Source: CAD feature listing. Evaluate the final solid. Frame: model axes, mm. A direction names the side the tool comes from. Give positions to 0.01 mm unless a question says otherwise; leave off trailing zeros. Order: outer loops, then holes, each group sorted by start corner. A loop starts at its lowest first (then second) coordinate and runs counter-clockwise, first axis right, second up. Notation, with made-up numbers: M 78,6.5 L 90,6.5 A17 cw 90,23.5 Z; hole C 82.25,-34 d2. An arc over 180 degrees is marked long. Answer as a JSON object with one key per item and string values. Group by question number.
1. Pull-direction query (Z, two-part tool) for faces 1 (the flat face through (21, -3, 6)), 2 (the flat face through (-12.5, -3, -28)), 3 (the flat face through (25, -3, 21)); classes: +Z half, -Z half, draft (parallel to the pull), parting line (faces both ways), or undercut.
2. Pin query (flat end, axial travel): P1, Ø3, axis at y = -3.5, z = -26.5, coming from the -X side; P2, Ø3, axis at x = -5.5, y = -2, coming from the -Z side; P3, Ø1.9, axis at x = 24.75, z = 5, coming from the +Y side. Return the tip coordinate at first contact, or that it passes through.
3. Section query B-B (z = -5). Output: boundary loops of the cut face in (x, y), plus the area to 3 significant figures.
4. Section query A-A (x = -10.5). Output: boundary loops of the cut face in (y, z).
5. Section query D-D (y = -4.95). Count the separate pieces of the cut face and the enclosed holes in it, plus the area to 3 significant figures.
6. Set-up query: faces 4 (the flat face through (-29, -3, -24.5)), 5 (the flat face through (27.5, -3, -28)), 6 (the flat face through (17.553, -3, 24)), 7 (the flat face through (21, -3, -6)). Return all of +Z, -Z, +X, -X, +Y, -Y with unobstructed straight access to the full face (end or side cutting, diameter ignored); none if empty.
7. Section query C-C (x = -24.75). Output: boundary loops of the cut face in (y, z).
8. Material intervals for L1, parallel to Z at x = 24.75, y = -1.75; L2, parallel to Z at x = 13, y = -3.7; L3, parallel to Z at x = -4, y = -4.5, sorted ascending. Write a range as [from, to].
from build123d import *

# Parameters (mm, degrees)
ESBO_O1_R                = 1.6
RESSALTO_EXTRUS_O1_DEPTH = 6


with BuildPart() as part:
    # Esboço1 → Ressalto-extrusão1 (new body)
    with BuildSketch(Plane.XZ.offset(6)):
        with BuildLine():
            Line((2.55259, 21), (-26.35, 21))
            ThreePointArc((-26.35, 21), (-29.885533906, 19.535533906), (-31.35, 16))
            Line((-31.35, 16), (-31.35, -24.5))
            Line((-31.35, -24.5), (-27.5, -24.5))
            Line((-27.5, -24.5), (-27.5, -30.5))
            Line((-27.5, -30.5), (-12.5, -30.5))
            Line((-12.5, -30.5), (-12.5, -24.5))
            Line((-12.5, -24.5), (12.5, -24.5))
            Line((12.5, -24.5), (12.5, -30.5))
            Line((12.5, -30.5), (27.5, -30.5))
            Line((27.5, -30.5), (27.5, -24.5))
            Line((27.5, -24.5), (31.35, -24.5))
            Line((31.35, -24.5), (31.35, 21))
            Line((31.35, 21), (17.55259, 21))
            Line((17.55259, 21), (17.55259, 27))
            Line((17.55259, 27), (2.55259, 27))
            Line((2.55259, 27), (2.55259, 21))
        make_face()
        with Locations((24.75, 5)):
            Circle(ESBO_O1_R, mode=Mode.SUBTRACT)
        with Locations((24.75, -5)):
            Circle(ESBO_O1_R, mode=Mode.SUBTRACT)
        with Locations((-24.75, 5)):
            Circle(ESBO_O1_R, mode=Mode.SUBTRACT)
        with Locations((-24.75, -5)):
            Circle(ESBO_O1_R, mode=Mode.SUBTRACT)
        Polygon((-26.35, 1.5), (-21, 1.5), (-21, 11), (21, 11), (21, 1.5), (26.35, 1.5), (26.35, -1.5), (21, -1.5), (21, -11), (-21, -11), (-21, -1.5), (-26.35, -1.5), align=None, mode=Mode.SUBTRACT)
    extrude(amount=-RESSALTO_EXTRUS_O1_DEPTH)


solid = part.part
Answer sheet:
{
 "1": {"face 1": "undercut", "face 2": "draft", "face 3": "+Z half"},
 "2": {"P1": "x = -27.5", "P2": "z = -24.5", "P3": "through"},
 "3": {"outline": "M -31.35,-6 L -26.35,-6 L -26.35,0 L -31.35,0 Z; M -23.15,-6 L -21,-6 L -21,0 L -23.15,0 Z; M 21,-6 L 23.15,-6 L 23.15,0 L 21,0 Z; M 26.35,-6 L 31.35,-6 L 31.35,0 L 26.35,0 Z", "area": "85.8 mm^2"},
 "4": {"outline": "M -6,-24.5 L 0,-24.5 L 0,-11 L -6,-11 Z; M -6,11 L 0,11 L 0,21 L -6,21 Z"},
 "5": {"separate pieces": "1", "enclosed holes": "5", "area": "2,130 mm^2"},
 "6": {"face 4": "-Z, -X, +Y, -Y", "face 5": "-Z, +X, +Y, -Y", "face 6": "+Z, +X, +Y, -Y", "face 7": "+Y, -Y"},
 "7": {"outline": "M -6,-30.5 L 0,-30.5 L 0,-6.6 L -6,-6.6 Z; M -6,-3.4 L 0,-3.4 L 0,-1.5 L -6,-1.5 Z; M -6,1.5 L 0,1.5 L 0,3.4 L -6,3.4 Z; M -6,6.6 L 0,6.6 L 0,21 L -6,21 Z"},
 "8": {"L1": "[-30.5, -6.6], [-3.4, -1.5], [1.5, 3.4], [6.6, 21]", "L2": "[-30.5, -11], [11, 27]", "L3": "[-24.5, -11], [11, 21]"}
}
